Geometry: see drawing. Coordinates: mm, zero at the bounding-box minimum. A direction names the side the tool comes from. Coordinates: 2 decimals unless noted, no trailing zeros. Order: outer loops, then holes, each group sorted by start corner. A loop starts at its lowest first (then second) coordinate and runs counter-clockwise, first axis right, second up.
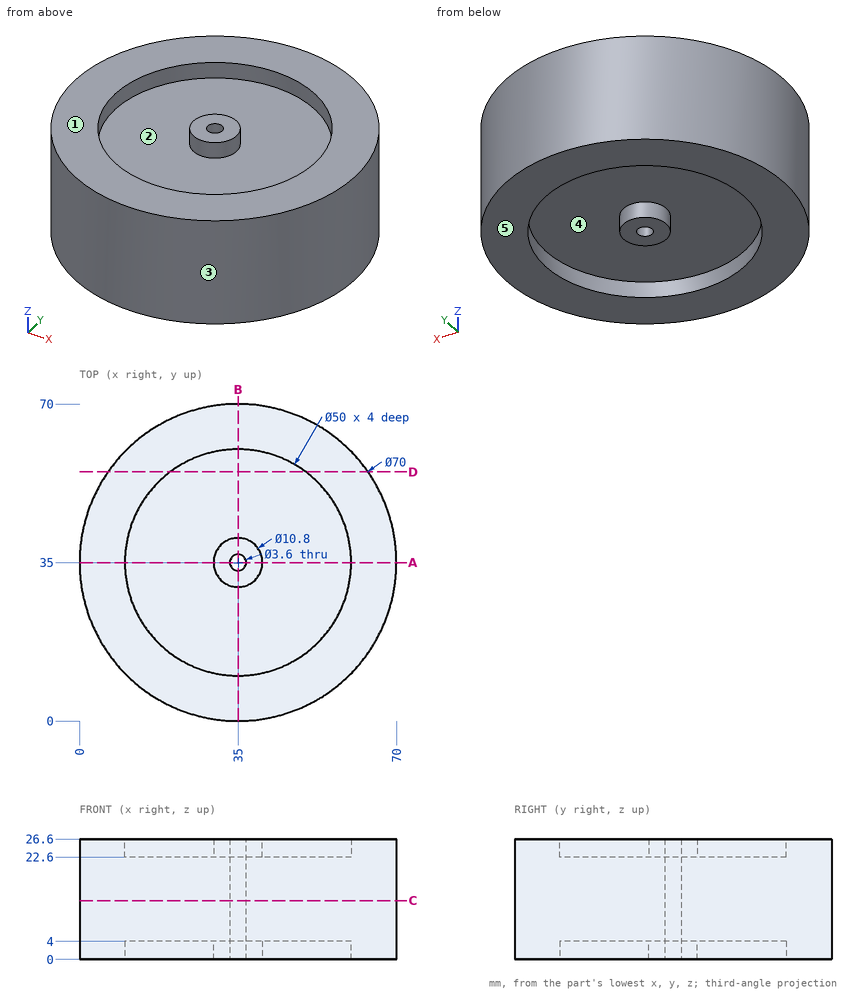
Item 1: Cut plane C-C on z = 13. Return loops of the section in (x, y), then the cut area to 3 significant figures.
Response values:
outline: circle Ø70 at (35, 35); hole circle Ø3.6 at (35, 35)
area: 3,840 mm2
Item 2: Draft query along X for the marked faces 3, 4 and 5. Return one class per face: pulls with the +X half, pulls with the -X half, needs draft (parallel to the pull), parting line crosses it, or undercut.
Response values:
face 3: parting line crosses it
face 4: undercut
face 5: needs draft
Item 3: Ray query, probe 1 along Y at (x, z) = (35, 25.3); probe 2 along Y at (x, z) = (35, 7.75); probe 3 along Z at (x, y) = (38, 53). Return the intervals inside material, ascending.
Response values:
probe 1: y = 0 to 10, 29.6 to 33.2, 36.8 to 40.4, 60 to 70
probe 2: y = 0 to 33.2, 36.8 to 70
probe 3: z = 4 to 22.6
Item 4: Access query for the marked faces 1 and 2. Directions: +Z, -Z, +X, -X, +Y, -Y. A direction counts if a zero-diameter tool reaches every point of the face in a straight line with its end or side. Return the directions, or none.
Response values:
face 1: +Z, +X, -X, +Y, -Y
face 2: +Z
Item 5: Pin query (flat end, axial travel): pin 1 Ø10 at (y, z) = (59.5, 23.5) entering from +X; pin 2 Ø1 at (x, z) = (48, 19) entering from +Y; pin 3 Ø5 at (x, z) = (28.5, 3) entering from -Y. Return the tip coordinate at first contact, or that it passes through.
Response values:
pin 1: stops at x = 64.06
pin 2: stops at y = 67.69
pin 3: stops at y = 0.23
Item 6: Cut plane D-D on y = 55. Return loops of the section in (x, z), then the cut area to 3 significant figures.
Response values:
outline: (6.28, 0) - (20, 0) - (20, 4) - (50, 4) - (50, 0) - (63.72, 0) - (63.72, 26.6) - (50, 26.6) - (50, 22.6) - (20, 22.6) - (20, 26.6) - (6.28, 26.6) - close
area: 1,290 mm2
Item 7: Cut plane A-A on y = 35. Return loops of the section in (x, z), then the cut area to 3 significant figures.
Response values:
outline: (0, 0) - (10, 0) - (10, 4) - (29.6, 4) - (29.6, 0) - (33.2, 0) - (33.2, 26.6) - (29.6, 26.6) - (29.6, 22.6) - (10, 22.6) - (10, 26.6) - (0, 26.6) - close; (36.8, 0) - (40.4, 0) - (40.4, 4) - (60, 4) - (60, 0) - (70, 0) - (70, 26.6) - (60, 26.6) - (60, 22.6) - (40.4, 22.6) - (40.4, 26.6) - (36.8, 26.6) - close
area: 1,450 mm2
